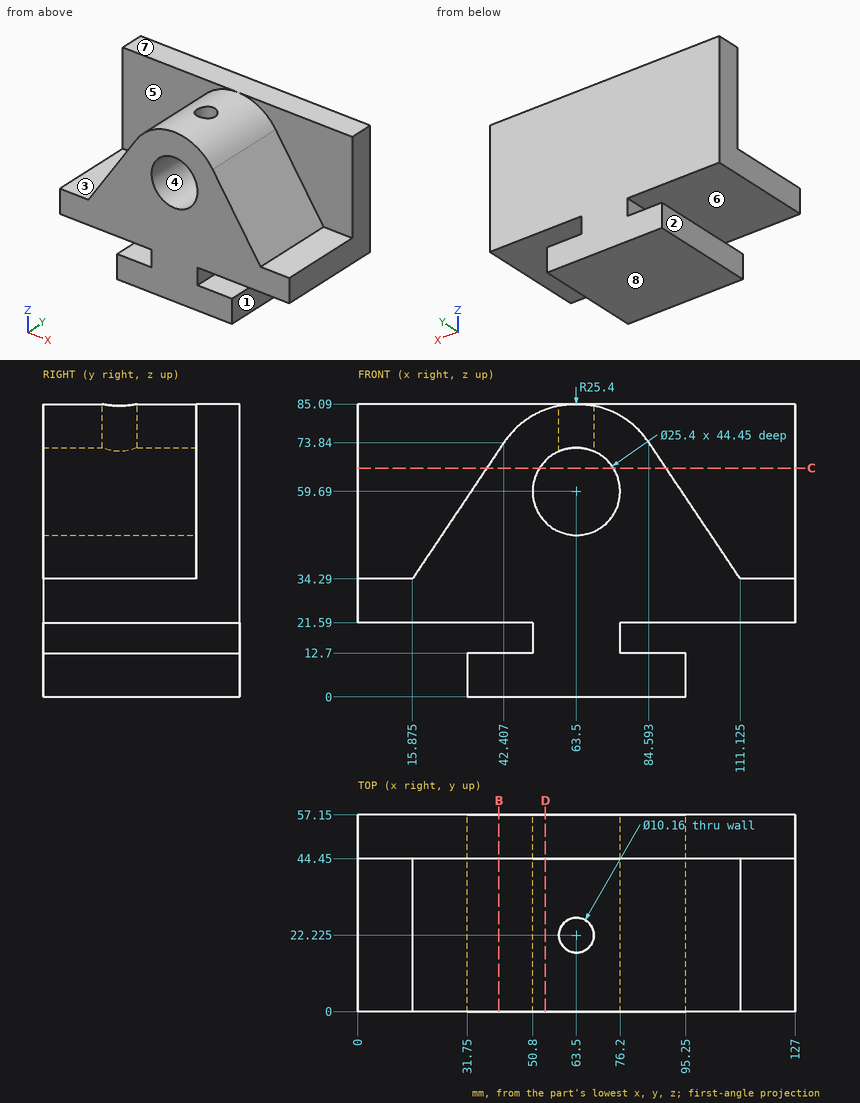
Geometry: see drawing. Coordinates: mm, zero at the bounding-box minimum. A direction names the side the tool comes from. Coordinates: 2 decimals unless noted, no trailing zeros. Order: outer loops, then holes, each group sorted by start corner. A loop starts at its lowest first (then second) coordinate and runs counter-clockwise, first axis right, second up. Notation, with made-up numbers: M -17,3 L 21,3 A23 ccw 21,22 Z; hole C 2.5,5 d8. An arc over 180 degrees is marked long. Answer in a Markdown table with one row per item. Add a question column.
Q1. Reachability of the marked faces 1, 2, 3 and 4 from +Z, -Z, +X, -X, +Y, -Y: full face, straight path, thin tool, end or side. Return the list, or none.
Q2. Line query: L1, parallel to Y at x = 63, z = 79; L2, parallel to Z at x = 63.5, y = 28; L3, parallel to Z at x = 43.5, y = 45.5. Output: solid intervals per line, ascending.
Q3. Section query C-C on z = 66.5. Return the cut outline in (x, y).
Q4. Mould query, pull axis Z, two halves, no side actions, for the marked faces 5, 6, 7 and 8. Classes: released by +Z, released by -Z, zero draft, split by the parting line, or undercut.
Q5. Section query D-D on x = 54.5. Return the cut outline in (y, z), and give its area (3 significant figures).
Q6. Section query B-B on x = 41. Return the cut outline in (y, z).
Q7. Contact query for flat-ended pins moving along their axis: P1, Ø3, axis at y = 20, z = 33.5, coming from the -X side; P2, Ø5.5, axis at x = 89.5, y = 21.5, coming from the +Z side (1 decimal); P3, Ø9.5, axis at x = 36.5, y = 14.5, coming from the +Z side (1 decimal); P4, Ø17.5, axis at x = 8, y = 30.5, coming from the +Z side (1 decimal). Output: stop coordinate, or through.
Completed:
| question | item | result |
|---|---|---|
| 1 | face 1 | -Z, +X, +Y, -Y |
| 1 | face 2 | -Z, -X, +Y, -Y |
| 1 | face 3 | +Z, -X, -Y |
| 1 | face 4 | -Y |
| 2 | L1 | y = 0 to 17.17, 27.28 to 57.15 |
| 2 | L2 | z = 0 to 46.99, 72.39 to 85.09 |
| 2 | L3 | z = 0 to 12.7, 21.59 to 85.09 |
| 3 | outline | M 0,44.45 L 37.48,44.45 L 37.48,0 L 52.78,0 L 52.78,44.45 L 74.22,44.45 L 74.22,0 L 89.52,0 L 89.52,44.45 L 127,44.45 L 127,57.15 L 0,57.15 Z |
| 4 | face 5 | zero draft |
| 4 | face 6 | undercut |
| 4 | face 7 | released by +Z |
| 4 | face 8 | released by -Z |
| 5 | outline | M 0,0 L 57.15,0 L 57.15,85.09 L 44.45,85.09 L 44.45,83.44 L 0,83.44 L 0,68.65 L 44.45,68.65 L 44.45,50.73 L 0,50.73 Z |
| 5 | area | 3,990 mm2 |
| 6 | outline | M 0,0 L 57.15,0 L 57.15,12.7 L 0,12.7 Z; M 0,21.59 L 57.15,21.59 L 57.15,85.09 L 44.45,85.09 L 44.45,71.74 L 0,71.74 Z |
| 7 | P1 | stops at x = 0 |
| 7 | P2 | stops at z = 70.6 |
| 7 | P3 | stops at z = 72.1 |
| 7 | P4 | stops at z = 35.6 |
